Part model, mm, in its own coordinate system. A direction names the side the tool comes from. Coordinates: 2 decimals unless noted, no trailing zeros. Write each loop counter-clockwise with the first axis right and the second up, starting at its lowest first coordinate (ties: lowest second). Pieces come first, ordered by that corner, then holes. Notation, with made-up numbers: (76.25, -15) -> (107.25, -15) arc R22 ccw to (107.25, -2) -> close; hole circle Ø8 at (88, 15). An arc over 180 degrees is marked (long way). Write item = value, one per line. Start each with the question number.
Q1. Pull direction X, two halves, no side cores. Call faces 3 (the flat face through (-25.4, -0.2, 0.5)), 4 (the flat face through (-14.493, -8.778, 0.507)), 5 (the flat face through (8.9, -12.35, 0.5)): released by +X, released by -X, zero draft, split by the parting line, or undercut.
Q2. Band-saw the part on A-A, the plane y = -9. List the corners of the cut face in (x, z).
Q3. Band-saw the part on C-C, the plane x = 17. List the corners of the cut face in (y, z).
Q4. Tool access for faces 1 (the flat face through (0, 0, 0)), 2 (the flat face through (-9.419, -8.877, 0.507)): list every direction of +Z, -Z, +X, -X, +Y, -Y with a clear straight run to the whole face (end or side of a thin tool).
Q5. Pin check, flat tip, straight feed: P1, Ø8, axis at x = 4, y = 5.5, coming from the -Z side. Stop position of the tip, or through.
Q6. Band-saw the part on D-D, the plane x = -13. List the corners of the cut face in (y, z), plus the area to 3 significant figures.
Q7. Band-saw the part on B-B, the plane z = 0.45. List the corners of the cut face in (x, y), plus the area to 3 significant figures.
Q8. Probe line 1 (X direction, y = 6.25, z = 0.45); line 2 (X direction, y = -10, z = 0.5); line 3 (Y direction, x = -13.5, z = 0.4). List the from-to ranges inside material, lowest first.
from build123d import *

# Parameters (mm, degrees)
F0_W     = 50.8
F0_H     = 24.7
F1_DEPTH = 1
F2_R     = 1.5
F3_DEPTH = 33.2
F4_R     = 2.413572
F5_DEPTH = 25
F7_DEPTH = 25


with BuildPart() as f1:
    # F0 (on Top) → F1 (new body)
    with BuildSketch(Plane.XY):
        Rectangle(F0_W, F0_H)
    extrude(amount=F1_DEPTH)

    # F2 (on face) → F3 (cut)
    with BuildSketch(Plane.XY.offset(1)):
        with Locations((19.324599, -3.538307)):
            Circle(F2_R)
    extrude(amount=F3_DEPTH, mode=Mode.SUBTRACT)

    # F4 (on face) → F5 (cut)
    with BuildSketch(Plane.XY.offset(1)):
        with Locations((18.560736, 6.366691)):
            Circle(F4_R)
    extrude(amount=-F5_DEPTH, mode=Mode.SUBTRACT)

    # F6 (on face) → F7 (cut)
    with BuildSketch(Plane.XY.offset(1)):
        Polygon((-11.734784, -5.304768), (-17.328629, -12.35), (-7.167339, -12.35), align=None)
    extrude(amount=-F7_DEPTH, mode=Mode.SUBTRACT)


solid = f1.part
Ans:
q1.face_3 = released by -X
q1.face_4 = undercut
q1.face_5 = zero draft
q2.outline = (-25.4, 0) -> (-14.67, 0) -> (-14.67, 1) -> (-25.4, 1) -> close; (-9.34, 0) -> (25.4, 0) -> (25.4, 1) -> (-9.34, 1) -> close
q3.outline = (-12.35, 0) -> (4.53, 0) -> (4.53, 1) -> (-12.35, 1) -> close; (8.21, 0) -> (12.35, 0) -> (12.35, 1) -> (8.21, 1) -> close
q4.face_1 = -Z, +X, -X, +Y, -Y
q4.face_2 = +Z, -Z, -Y
q5.P1 = 0
q6.outline = (-6.9, 0) -> (12.35, 0) -> (12.35, 1) -> (-6.9, 1) -> close
q6.area = 19.2 mm2
q7.outline = (-25.4, -12.35) -> (-17.33, -12.35) -> (-11.73, -5.3) -> (-7.17, -12.35) -> (25.4, -12.35) -> (25.4, 12.35) -> (-25.4, 12.35) -> close; hole circle Ø4.83 at (18.56, 6.37)
q7.area = 1,200 mm2
q8.line_1 = -25.4 to 16.15, 20.97 to 25.4
q8.line_2 = -25.4 to -15.46, -8.69 to 25.4
q8.line_3 = -7.53 to 12.35
